Here's the drawing with two shaded views (mm, measured from the low corner). I have some questions. A direction names the side the tool comes from. Round coordinates to 2 decimals unless told otherwise and drop trailing zeros. Write each loop counter-clockwise with the first axis right and the second up, starting at its lowest first coordinate (ties: lowest second). Pieces come first, ordered by that corner, then holes. Notation, with made-up numbers: M 55,19 L 94,19 A21 cw 94,35 Z; hole C -28,32 d7. An arc over 180 degrees is marked long. Write item = value, one per line. Start each with the question number.
(1) I want a section at D-D (x = 46.5). List the corners of the cut face in (y, z) for me, and give its area (3 significant figures).
(2) If we mould it in two halves opening along X, with no side actions, what happens to the marked faces 1, 2 and 3? For each: released by +X, released by -X, zero draft, split by the parting line, or undercut.
(3) Will these pins go through, and if not, where does the flat tip stop? pin 1 Ø8 at (y, z) = (13.5, 9.5) entering from +X; pin 2 Ø4 at (y, z) = (12, 26.5) entering from -X; pin 3 Ø5 at (y, z) = (13.5, 10) entering from +X; pin 4 Ø5 at (x, y) = (4.5, 14.5) entering from +Z.
(4) I need wall thicknesses on line 1 along X through (y, z) = (9.25, 3); line 2 along Y through (x, z) = (54, 1.6); line 3 along Y through (x, z) = (30, 23). Which ranges of each line are inside material? Lowest first, please.
(5) I want a section at B-B (y = 10). List the corners of the cut face in (x, z) for me, and give its area (3 significant figures).
(6) I want a section at C-C (z = 29.5). List the corners of the cut face in (x, y) for me.
(7) I want a section at A-A (x = 54). List the corners of the cut face in (y, z) for me, and give its area (3 significant figures).
(8) On a 3-axis mill with a long thin cutter (end or side, diameter ignored), from which of +Z, -Z, +X, -X, +Y, -Y can I reach the whole of each face in a straight line? I mean the marked faces 4, 5 and 6. Say none if no direction works.
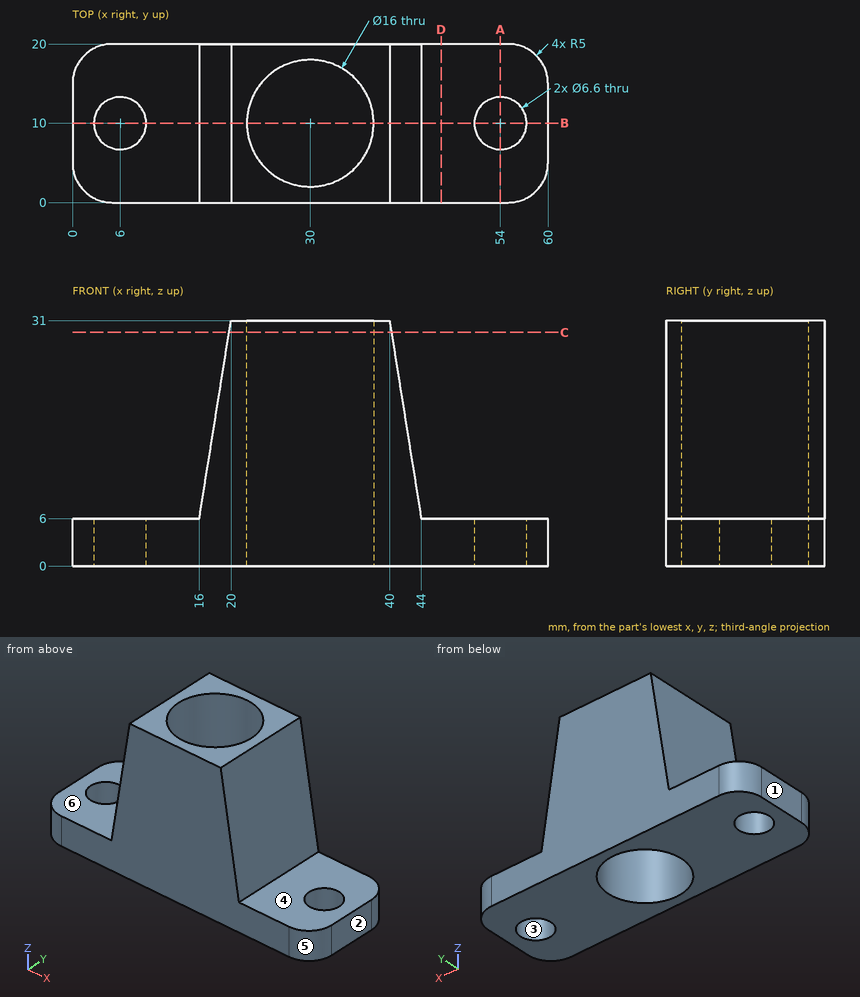
Returned:
q1.outline = M 0,0 L 20,0 L 20,6 L 0,6 Z
q1.area = 120 mm²
q2.face_1 = released by -X
q2.face_2 = released by +X
q2.face_3 = undercut
q3.pin_1 = 60
q3.pin_2 = 18.96
q3.pin_3 = 43.76
q3.pin_4 = 6
q4.line_1 = 0 to 2.79, 9.21 to 22.04, 37.96 to 50.79, 57.21 to 60
q4.line_2 = 0 to 6.7, 13.3 to 20
q4.line_3 = 0 to 2, 18 to 20
q5.outline = M 0,0 L 2.7,0 L 2.7,6 L 0,6 Z; M 9.3,0 L 22,0 L 22,31 L 20,31 L 16,6 L 9.3,6 Z; M 38,0 L 50.7,0 L 50.7,6 L 44,6 L 40,31 L 38,31 Z; M 57.3,0 L 60,0 L 60,6 L 57.3,6 Z
q5.area = 385 mm²
q6.outline = M 19.76,0 L 40.24,0 L 40.24,20 L 19.76,20 Z; hole C 30,10 d16
q7.outline = M 0,0 L 6.7,0 L 6.7,6 L 0,6 Z; M 13.3,0 L 20,0 L 20,6 L 13.3,6 Z
q7.area = 80.4 mm²
q8.face_4 = +Z, +X, +Y, -Y
q8.face_5 = +Z, -Z, +X, -Y
q8.face_6 = +Z, -X, +Y, -Y
